Verification items for the finished model (mm, model axes). A direction names the side the tool comes from. Give positions to 0.01 mm unless a question says otherwise; leave off trailing zeros. Loops run counter-clockwise (first coordinate to the right, second up) from the corner with the lowest first, then second, coordinate; pieces in that order, holes last. Notation, with made-up numbers: M 68,7 L 73,7 A16 cw 73,27 Z; hole C 39.25,-9.75 d10. An arc over 180 degrees is marked long. Answer in a Markdown table with one row per item.
```python
from build123d import *

# Parameters (mm, degrees)
SKETCH2_R           = 2.667
BOSS_EXTRUDE1_DEPTH = 5.08
FILLET1_R           = 1.27
FILLET2_R           = 0.762


with BuildPart() as part:
    # Sketch2 → Boss-Extrude1 (new body)
    with BuildSketch(Plane(origin=(104.932978861, 0, 0), x_dir=(0, 0, -1), z_dir=(1, 0, 0))):
        Polygon((-107.309772969, 81.573572085), (-107.309772969, 65.825572085), (-107.309772969, 60.745572085), (-107.309772969, 44.235572085), (-103.499772969, 44.235572085), (-103.499772969, 46.775572085), (-103.499772969, 71.667572085), (-97.657772969, 71.667572085), (-97.657772969, 46.775572085), (-97.657772969, 44.235572085), (-91.561772969, 44.235572085), (-91.561772969, 46.775572085), (-91.561772969, 71.667572085), (-75.559772969, 71.667572085), (-75.559772969, 46.775572085), (-75.559772969, 44.235572085), (-71.749772969, 44.235572085), (-71.749772969, 70.905572085), (-61.081772969, 70.905572085), (-61.081772969, 81.573572085), align=None)
        with Locations((-66.415772969, 76.239572085)):
            Circle(SKETCH2_R, mode=Mode.SUBTRACT)
    extrude(amount=BOSS_EXTRUDE1_DEPTH)

    # Fillet1
    fillet1_edges = [part.edges().sort_by_distance(p)[0] for p in [
        (107.472978861, 81.573572085, 61.081772969),
        (107.472978861, 70.905572085, 61.081772969),
        (107.472978861, 70.905572085, 71.749772969),
        (107.472978861, 44.235572085, 71.749772969),
        (107.472978861, 44.235572085, 75.559772969),
        (107.472978861, 71.667572085, 75.559772969),
        (107.472978861, 71.667572085, 91.561772969),
        (107.472978861, 44.235572085, 91.561772969),
        (107.472978861, 44.235572085, 97.657772969),
        (107.472978861, 71.667572085, 97.657772969),
        (107.472978861, 71.667572085, 103.499772969),
        (107.472978861, 44.235572085, 103.499772969),
        (107.472978861, 44.235572085, 107.309772969),
        (107.472978861, 81.573572085, 107.309772969),
    ]]
    fillet(fillet1_edges, radius=FILLET1_R)

    # Fillet2
    fillet2_edges = [part.edges().sort_by_distance(p)[0] for p in [
        (110.012978861, 70.533597697, 71.377798581),
        (110.012978861, 57.570572085, 71.749772969),
        (110.012978861, 44.607546473, 72.121747356),
        (110.012978861, 44.235572085, 73.654772969),
        (110.012978861, 44.607546473, 75.187798581),
        (110.012978861, 57.951572085, 75.559772969),
        (110.012978861, 71.295597697, 75.931747356),
        (110.012978861, 71.667572085, 83.560772969),
        (110.012978861, 71.295597697, 91.189798581),
        (110.012978861, 57.951572085, 91.561772969),
        (110.012978861, 44.607546473, 91.933747356),
        (110.012978861, 44.235572085, 94.609772969),
        (110.012978861, 44.607546473, 97.285798581),
        (110.012978861, 57.951572085, 97.657772969),
        (110.012978861, 71.295597697, 98.029747356),
        (110.012978861, 71.667572085, 100.578772969),
        (110.012978861, 71.295597697, 103.127798581),
        (110.012978861, 57.951572085, 103.499772969),
        (110.012978861, 44.607546473, 103.871747356),
        (110.012978861, 44.235572085, 105.404772969),
        (110.012978861, 44.607546473, 106.937798581),
        (110.012978861, 62.904572085, 107.309772969),
        (110.012978861, 81.201597697, 106.937798581),
        (110.012978861, 81.573572085, 84.195772969),
        (110.012978861, 81.201597697, 61.453747356),
        (110.012978861, 76.239572085, 61.081772969),
        (110.012978861, 71.277546473, 61.453747356),
        (110.012978861, 70.905572085, 66.415772969),
    ]]
    fillet(fillet2_edges, radius=FILLET2_R)


solid = part.part
```
Item 1: Tool access check on faces 1 (the flat face through (110.013, 67, 94)), 2 (the flat face through (107, 70.906, 66)), 3 (the flat face through (107, 58, 75.56)). Record the directions out of +Z, -Z, +X, -X, +Y, -Y that give a thin tool (end or side, any length) a straight path to the whole face; none if there is none.
Reported:
| item | result |
|---|---|
| face 1 | +Z, -Z, +X, +Y, -Y |
| face 2 | -Z, +X, -X, -Y |
| face 3 | +X, -X, -Y |
Item 2: Sectioned sample at B-B (z = 67). Record the cut outline in (x, y), and give its area (3 significant figures).
Reported:
| item | result |
|---|---|
| outline | M 104.93,70.91 L 109.25,70.91 A0.76 ccw 110.01,71.67 L 110.01,73.64 L 104.93,73.64 Z; M 104.93,78.84 L 110.01,78.84 L 110.01,80.81 A0.76 ccw 109.25,81.57 L 104.93,81.57 Z |
| area | 27.5 mm^2 |
Item 3: Sectioned sample at A-A (y = 62.5). Record the cut outline in (x, z), and give its area (3 significant figures).
Reported:
| item | result |
|---|---|
| outline | M 104.93,71.75 L 109.25,71.75 A0.76 ccw 110.01,72.51 L 110.01,74.8 A0.76 ccw 109.25,75.56 L 104.93,75.56 Z; M 104.93,91.56 L 109.25,91.56 A0.76 ccw 110.01,92.32 L 110.01,96.9 A0.76 ccw 109.25,97.66 L 104.93,97.66 Z; M 104.93,103.5 L 109.25,103.5 A0.76 ccw 110.01,104.26 L 110.01,106.55 A0.76 ccw 109.25,107.31 L 104.93,107.31 Z |
| area | 68.9 mm^2 |
Item 4: Go/stop test with flat-tipped pins: pin 1 (2 mm diameter, centred on x = 106.5, y = 58.5, fed in from -Z); pin 2 (1.3 mm diameter, centred on x = 108, z = 86.5, fed in from -Y); pin 3 (8 mm diameter, centred on y = 67, z = 83, fed in from +X); pin 4 (7 mm diameter, centred on y = 76.24, z = 66.42, fed in from -X). Record where each tip stops, or that it passes through.
Reported:
| item | result |
|---|---|
| pin 1 | stops at z = 71.75 |
| pin 2 | stops at y = 71.67 |
| pin 3 | passes through |
| pin 4 | stops at x = 104.93 |
Item 5: Sectioned sample at D-D (z = 87). Record the cut outline in (x, y).
Reported:
| item | result |
|---|---|
| outline | M 104.93,71.67 L 109.25,71.67 A0.76 ccw 110.01,72.43 L 110.01,80.81 A0.76 ccw 109.25,81.57 L 104.93,81.57 Z |
Item 6: Scan lines: L1, parallel to Z at x = 106.6, y = 55; L2, parallel to Y at x = 108.95, z = 63; L3, parallel to Z at x = 106.1, y = 70.5. Record each from-to range of solid material in increasing order. Write a range as [from, to].
Reported:
| item | result |
|---|---|
| L1 | z = [71.75, 75.56], [91.56, 97.66], [103.5, 107.31] |
| L2 | y = [70.91, 81.57] |
| L3 | z = [71.41, 75.56], [91.56, 97.66], [103.5, 107.31] |
